from build123d import *

# Parameters (mm, degrees)
F1_DEPTH = 1
F2_DEPTH = 5
F3_DEPTH = 7


with BuildPart() as f1:
    # F0 (on Top) → F1 (new body)
    with BuildSketch(Plane.XY):
        with BuildLine():
            Line((-29, 44), (-29, 0))
            Line((-29, 0), (-29, -44))
            ThreePointArc((-29, -44), (-27.535534, -47.535534), (-24, -49))
            Line((-24, -49), (0, -49))
            Line((0, -49), (24, -49))
            ThreePointArc((24, -49), (27.535534, -47.535534), (29, -44))
            Line((29, -44), (29, 0))
            Line((29, 0), (29, 44))
            ThreePointArc((29, 44), (27.535534, 47.535534), (24, 49))
            Line((24, 49), (0, 49))
            Line((0, 49), (-24, 49))
            ThreePointArc((-24, 49), (-27.535534, 47.535534), (-29, 44))
        make_face()
    extrude(amount=F1_DEPTH)

    # F0 (on Top) → F2 (join)
    with BuildSketch(Plane.XY):
        with BuildLine():
            Line((-30, 45), (-30, 0))
            Line((-30, 0), (-30, -45))
            ThreePointArc((-30, -45), (-28.535534, -48.535534), (-25, -50))
            Line((-25, -50), (25, -50))
            ThreePointArc((25, -50), (28.535534, -48.535534), (30, -45))
            Line((30, -45), (30, 0))
            Line((30, 0), (30, 45))
            ThreePointArc((30, 45), (28.535534, 48.535534), (25, 50))
            Line((25, 50), (-25, 50))
            ThreePointArc((-25, 50), (-28.535534, 48.535534), (-30, 45))
        make_face()
        with BuildLine():
            Line((-29, -44), (-29, 0))
            Line((-29, 0), (-29, 44))
            ThreePointArc((-29, 44), (-27.535534, 47.535534), (-24, 49))
            Line((-24, 49), (0, 49))
            Line((0, 49), (24, 49))
            ThreePointArc((24, 49), (27.535534, 47.535534), (29, 44))
            Line((29, 44), (29, 0))
            Line((29, 0), (29, -44))
            ThreePointArc((29, -44), (27.535534, -47.535534), (24, -49))
            Line((24, -49), (0, -49))
            Line((0, -49), (-24, -49))
            ThreePointArc((-24, -49), (-27.535534, -47.535534), (-29, -44))
        make_face(mode=Mode.SUBTRACT)
        with BuildLine():
            Line((-29, 44), (-29, 0))
            Line((-29, 0), (-29, -44))
            ThreePointArc((-29, -44), (-27.535534, -47.535534), (-24, -49))
            Line((-24, -49), (0, -49))
            Line((0, -49), (24, -49))
            ThreePointArc((24, -49), (27.535534, -47.535534), (29, -44))
            Line((29, -44), (29, 0))
            Line((29, 0), (29, 44))
            ThreePointArc((29, 44), (27.535534, 47.535534), (24, 49))
            Line((24, 49), (0, 49))
            Line((0, 49), (-24, 49))
            ThreePointArc((-24, 49), (-27.535534, 47.535534), (-29, 44))
        make_face()
    extrude(amount=-F2_DEPTH)

    # F1_face (on face) → F3 (join)
    with BuildSketch(Plane.XY.offset(1)):
        with BuildLine():
            Line((-29, 44), (-29, -44))
            ThreePointArc((-29, -44), (-27.535534, -47.535534), (-24, -49))
            Line((-24, -49), (24, -49))
            ThreePointArc((24, -49), (27.535534, -47.535534), (29, -44))
            Line((29, -44), (29, 44))
            ThreePointArc((29, 44), (27.535534, 47.535534), (24, 49))
            Line((24, 49), (-24, 49))
            ThreePointArc((-24, 49), (-27.535534, 47.535534), (-29, 44))
        make_face()
    extrude(amount=-F3_DEPTH)


solid = f1.part
Verification items for the finished model (mm, model axes). A direction names the side the tool comes from. Coordinates: 2 decimals unless noted, no trailing zeros. Use CSV: the item, a comma, the result in double quotes.
Q1. Thickness scan on line 1 along X through (y, z) = (-38, -5.5); line 2 along Y through (x, z) = (0, -5.25). Record the ranges inside material, lowest first. Write a range as [from, to].
Computed values:
line 1,"[-29, 29]"
line 2,"[-49, 49]"
Q2. Go/stop test with flat-tipped pins: P1, Ø0.8, axis at x = -8.5, z = 0.5, coming from the -Y side; P2, Ø0.8, axis at x = -11.5, z = 0.5, coming from the +Y side. Record where each tip stops, or that it passes through.
Computed values:
P1,"y = -49"
P2,"y = 49"
Q3. Set-up check for faces 1 (the cylindrical face through (-27.57, -47.5, -5.49)), 2 (the cylindrical face through (-27.5, 47.57, -5.49)), 3 (the cylindrical face through (27.5, -47.57, -5.49)), 4 (the cylindrical face through (-27.5, 47.57, 0.49)): record each of +Z, -Z, +X, -X, +Y, -Y from which the full face is reachable in a straight line by a thin tool's end or side.
Computed values:
face 1,"-Z, -X, -Y"
face 2,"-Z, -X, +Y"
face 3,"-Z, +X, -Y"
face 4,"+Z, -X, +Y"
